from build123d import *

# Parameters (mm, degrees)
F1_DEPTH = 9.144


with BuildPart() as f1:
    # F0 (on Top) → F1 (new body)
    with BuildSketch(Plane.XY):
        Polygon((38.1, 0), (25.4, 0), (25.4, -9.144), (9.144, -9.144), (9.144, -19.05), (0, -19.05), (0, -31.75), (9.144, -31.75), (9.144, -44.45), (0, -44.45), (0, -57.15), (9.144, -57.15), (9.144, -69.85), (0, -69.85), (0, -82.55), (9.144, -82.55), (9.144, -95.25), (0, -95.25), (0, -107.95), (9.144, -107.95), (9.144, -120.65), (0, -120.65), (0, -133.35), (9.144, -133.35), (9.144, -146.05), (0, -146.05), (0, -158.75), (9.144, -158.75), (9.144, -171.45), (0, -171.45), (0, -184.15), (9.144, -184.15), (9.144, -196.85), (0, -196.85), (0, -209.55), (9.144, -209.55), (9.144, -219.456), (25.4, -219.456), (25.4, -228.6), (38.1, -228.6), (38.1, -219.456), (50.8, -219.456), (50.8, -228.6), (63.5, -228.6), (63.5, -219.456), (76.2, -219.456), (76.2, -228.6), (88.9, -228.6), (88.9, -219.456), (101.6, -219.456), (101.6, -228.6), (114.3, -228.6), (114.3, -219.456), (127, -219.456), (127, -228.6), (139.7, -228.6), (139.7, -219.456), (152.4, -219.456), (152.4, -228.6), (165.1, -228.6), (165.1, -219.456), (177.8, -219.456), (177.8, -228.6), (190.5, -228.6), (190.5, -219.456), (203.2, -219.456), (203.2, -228.6), (215.9, -228.6), (215.9, -219.456), (228.6, -219.456), (228.6, -228.6), (241.3, -228.6), (241.3, -219.456), (254, -219.456), (254, -228.6), (266.7, -228.6), (266.7, -219.456), (282.956, -219.456), (282.956, -209.55), (292.1, -209.55), (292.1, -196.85), (282.956, -196.85), (282.956, -184.15), (292.1, -184.15), (292.1, -171.45), (282.956, -171.45), (282.956, -158.75), (292.1, -158.75), (292.1, -146.05), (282.956, -146.05), (282.956, -133.35), (292.1, -133.35), (292.1, -120.65), (282.956, -120.65), (282.956, -107.95), (292.1, -107.95), (292.1, -95.25), (282.956, -95.25), (282.956, -82.55), (292.1, -82.55), (292.1, -69.85), (282.956, -69.85), (282.956, -57.15), (292.1, -57.15), (292.1, -44.45), (282.956, -44.45), (282.956, -31.75), (292.1, -31.75), (292.1, -19.05), (282.956, -19.05), (282.956, -9.144), (266.7, -9.144), (266.7, 0), (254, 0), (254, -9.144), (241.3, -9.144), (241.3, 0), (228.6, 0), (228.6, -9.144), (215.9, -9.144), (215.9, 0), (203.2, 0), (203.2, -9.144), (190.5, -9.144), (190.5, 0), (177.8, 0), (177.8, -9.144), (165.1, -9.144), (165.1, 0), (152.4, 0), (152.4, -9.144), (139.7, -9.144), (139.7, 0), (127, 0), (127, -9.144), (114.3, -9.144), (114.3, 0), (101.6, 0), (101.6, -9.144), (88.9, -9.144), (88.9, 0), (76.2, 0), (76.2, -9.144), (63.5, -9.144), (63.5, 0), (50.8, 0), (50.8, -9.144), (38.1, -9.144), align=None)
    extrude(amount=F1_DEPTH)


solid = f1.part
Could you check a few things on this model? Use its own coordinates, in mm. A direction names the side the tool comes from. Round coordinates to 2 decimals unless told otherwise and drop trailing zeros. Loops run counter-clockwise (first coordinate to the right, second up) from the corner with the lowest first, then second, coordinate; pieces in that order, holes last. Notation, with made-up numbers: (12, -14) -> (17, -14) arc R20 cw to (17, 16) -> close; hole circle Ø4 at (-15, -32). An arc over 180 degrees is marked (long way). Use CSV: the item, a comma, the result in double quotes.
(1) If we mould it in two halves opening along Y, with no side actions, what happens to faces 5 (the flat face through (45, -9.144, 5)), 6 (the flat face through (9.144, -38, 5)), 7 (the flat face through (0, -25, 5))? For each: +Y half, -Y half, draft (parallel to the pull), parting line (faces both ways), or undercut.
Return value:
face 5,"+Y half"
face 6,"undercut"
face 7,"draft"
(2) For faces 1 (the flat face through (5, -184.15, 5)), 2 (the flat face through (287, -107.95, 5)), 3 (the flat face through (95, -9.144, 5)), 4 (the flat face through (275, -219.456, 5)), which set-ups out of +Z, -Z, +X, -X, +Y, -Y let a thin tool reach every point of the face, with its end or its side?
Return value:
face 1,"+Z, -Z, -X"
face 2,"+Z, -Z, +X"
face 3,"+Z, -Z, +Y"
face 4,"+Z, -Z, +X, -Y"
(3) Will these pins go through, and if not, where does the flat tip stop? pin 1 Ø2.5 at (y, z) = (-225.5, 5) entering from +X; pin 2 Ø2 at (y, z) = (-64.5, 6) entering from -X; pin 3 Ø4.5 at (y, z) = (-5.5, 3.5) entering from -X.
Return value:
pin 1,"stops at x = 266.7"
pin 2,"stops at x = 9.14"
pin 3,"stops at x = 25.4"
(4) Suppose I cut it at A-A on x = 20. Write out the boundary of the cut face in (y, z).
Return value:
outline,"(-219.46, 0) -> (-9.14, 0) -> (-9.14, 9.14) -> (-219.46, 9.14) -> close"
(5) Suppose I cut it at B-B on y = -142. Write out the boundary of the cut face in (x, z).
Return value:
outline,"(9.14, 0) -> (282.96, 0) -> (282.96, 9.14) -> (9.14, 9.14) -> close"
(6) If I drill on probe 1 along Y at (x, z) = (21, 6.75); probe 2 along X at (y, z) = (-41, 4.25), over which ranges is the centre line in solid material (lowest first)? Write a range as [from, to].
Return value:
probe 1,"y = [-219.46, -9.14]"
probe 2,"x = [9.14, 282.96]"
